```python
from build123d import *

# Parameters (mm, degrees)
PAD002_DEPTH = 0.35
PAD_DEPTH    = 2.55
CHAMFER_SIZE = 0.4
SKETCH003_R  = 0.503583
PAD003_DEPTH = 0.075
PAD001_DEPTH = 0.35


with BuildPart() as pad002:
    # Sketch002 → Pad002 (new body, symmetric)
    with BuildSketch(Plane.XZ.offset(-2)):
        Polygon((-3.1, 0), (-2.9, 0), (-2.4, 0.65), (2.4, 0.65), (2.9, 0), (3.1, 0), (3.1, 0.2), (3, 0.2), (2.5, 0.85), (-2.5, 0.85), (-3, 0.2), (-3.1, 0.2), align=None)
    extrude(amount=PAD002_DEPTH, both=True)


with BuildPart() as chamfer_body:
    # Sketch → Pad (new body, symmetric)
    with BuildSketch(Plane.XZ):
        Polygon((-2.25, 0.1), (2.25, 0.1), (2.3, 0.85), (2.25, 1.6), (-2.25, 1.6), (-2.3, 0.85), align=None)
    extrude(amount=PAD_DEPTH, both=True)

    # Chamfer
    chamfer_edges = [chamfer_body.edges().sort_by_distance(p)[0] for p in [
        (-2.25, 0, 1.6),
    ]]
    chamfer(chamfer_edges, length=CHAMFER_SIZE)


with BuildPart() as pad003:
    # Sketch003 → Pad003 (new body)
    with BuildSketch(Plane.XY.offset(1.55)):
        with Locations((-1.162023, 1.741391)):
            Circle(SKETCH003_R)
    extrude(amount=PAD003_DEPTH)


with BuildPart() as obj1:
    # Sketch001 → Pad001 (new body, symmetric)
    with BuildSketch(Plane.XZ.offset(2)):
        Polygon((-3.1, 0), (-2.9, 0), (-2.4, 0.65), (2.4, 0.65), (2.9, 0), (3.1, 0), (3.1, 0.2), (3, 0.2), (2.5, 0.85), (-2.5, 0.85), (-3, 0.2), (-3.1, 0.2), align=None)
    extrude(amount=PAD001_DEPTH, both=True)

    add(pad002.part)
    add(chamfer_body.part)
    add(pad003.part)


solid = obj1.part
```
Source: CAD feature listing. Evaluate the final solid. Frame: model axes, mm. Give positions to 0.01 mm unless a question says otherwise; leave off trailing zeros. Loops run counter-clockwise (first coordinate to the right, second up) from the corner with the lowest first, then second, coordinate; pieces in that order, holes last. Notation, with made-up numbers: (70.25, 77.25) -> (128.25, 77.25) arc R29 cw to (128.25, 110.25) -> close; hole circle Ø8 at (82, -1.75). An arc over 180 degrees is marked (long way). Use a Markdown table: item, result. Add a question column.
(1) Section query A-A (z = 0.5). Output: boundary loops of the cut face in (x, y).
(2) Section query B-B (y = 0.1). Output: boundary loops of the cut face in (x, z), then the cut area to 3 significant figures.
(3) Section query D-D (x = 1.25). Output: boundary loops of the cut face in (y, z).
(4) Section query C-C (x = -1.25). Output: boundary loops of the cut face in (y, z) (3 decimals).
(5) Pull-direction query (X, two-part tool) for faces 1 (the face through (0, 0, 0.1)), 2 (the face through (-1, 2, 1.625)); classes: +X half, -X half, draft (parallel to the pull), parting line (faces both ways), or undercut.
(6) Ray query, line 1 (Z direction, x = -0.75, y = 1.8) (3 decimals); line 2 (X direction, y = -0.4, z = 1.45); line 3 (X direction, y = 0.3, z = 0.8). Return the intervals inside material, ascending.
Checked values:
| question | item | result |
|---|---|---|
| 1 | outline | (-2.77, -2.35) -> (-2.52, -2.35) -> (-2.52, -1.65) -> (-2.77, -1.65) -> close; (-2.77, 1.65) -> (-2.52, 1.65) -> (-2.52, 2.35) -> (-2.77, 2.35) -> close; (-2.28, -2.55) -> (2.28, -2.55) -> (2.28, 2.55) -> (-2.28, 2.55) -> close; (2.52, -2.35) -> (2.77, -2.35) -> (2.77, -1.65) -> (2.52, -1.65) -> close; (2.52, 1.65) -> (2.77, 1.65) -> (2.77, 2.35) -> (2.52, 2.35) -> close |
| 2 | outline | (-2.3, 0.85) -> (-2.25, 0.1) -> (2.25, 0.1) -> (2.3, 0.85) -> (2.25, 1.6) -> (-1.85, 1.6) -> (-2.28, 1.2) -> close |
| 2 | area | 6.75 mm^2 |
| 3 | outline | (-2.55, 0.1) -> (2.55, 0.1) -> (2.55, 1.6) -> (-2.55, 1.6) -> close |
| 4 | outline | (-2.55, 0.1) -> (2.55, 0.1) -> (2.55, 1.6) -> (2.237, 1.6) -> (2.237, 1.625) -> (1.246, 1.625) -> (1.246, 1.6) -> (-2.55, 1.6) -> close |
| 5 | face 1 | undercut |
| 5 | face 2 | draft |
| 6 | line 1 | 0.1 to 1.625 |
| 6 | line 2 | -2.01 to 2.26 |
| 6 | line 3 | -2.3 to 2.3 |
